```python
from build123d import *

# Parameters (mm, degrees)
F1_DEPTH = 5.08
F2_R     = 3.175
F4_DEPTH = 12.7
F5_W     = 14.224
F5_H     = 14.224
F6_DEPTH = 43.7134


with BuildPart() as f1:
    # F0 (on Front) → F1 (new body)
    with BuildSketch(Plane.XZ):
        with BuildLine():
            Line((9.525, 12.7), (-9.525, 12.7))
            ThreePointArc((-9.525, 12.7), (-11.770064, 11.770064), (-12.7, 9.525))
            Line((-12.7, 9.525), (-12.7, -9.525))
            ThreePointArc((-12.7, -9.525), (-11.770064, -11.770064), (-9.525, -12.7))
            Line((-9.525, -12.7), (9.525, -12.7))
            ThreePointArc((9.525, -12.7), (11.770064, -11.770064), (12.7, -9.525))
            Line((12.7, -9.525), (12.7, 9.525))
            ThreePointArc((12.7, 9.525), (11.770064, 11.770064), (9.525, 12.7))
        make_face()
    extrude(amount=F1_DEPTH)

    # F2
    f2_edges = [f1.edges().sort_by_distance(p)[0] for p in [
        (12.7, -5.08, 0),
    ]]
    fillet(f2_edges, radius=F2_R)

    # F3 (on face) → F4 (join)
    with BuildSketch(Plane(origin=(0, 0, 0), x_dir=(-1, 0, 0), z_dir=(0, 1, 0))):
        with BuildLine():
            ThreePointArc((9.652, 8.636), (9.35442, 9.35442), (8.636, 9.652))
            Line((8.636, 9.652), (-8.636, 9.652))
            ThreePointArc((-8.636, 9.652), (-9.35442, 9.35442), (-9.652, 8.636))
            Line((-9.652, 8.636), (-9.652, -8.636))
            ThreePointArc((-9.652, -8.636), (-9.35442, -9.35442), (-8.636, -9.652))
            Line((-8.636, -9.652), (8.636, -9.652))
            ThreePointArc((8.636, -9.652), (9.35442, -9.35442), (9.652, -8.636))
            Line((9.652, -8.636), (9.652, 8.636))
        make_face()
    extrude(amount=F4_DEPTH)

    # F5 (on face) → F6 (cut)
    with BuildSketch(Plane(origin=(0, 0, 0), x_dir=(-1, 0, 0), z_dir=(0, 1, 0))):
        Rectangle(F5_W, F5_H)
    extrude(amount=F6_DEPTH, mode=Mode.SUBTRACT)


solid = f1.part
```
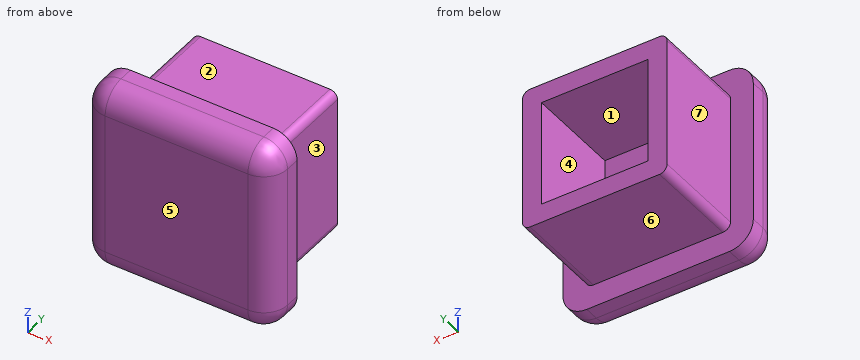
For this review, take the finished solid that the model builds, in its own axes (mm). Face numbers are marked on the shaded views. A direction names the side the tool comes from. Round coordinates to 2 decimals unless told otherwise and drop trailing zeros. Order: outer loops, then holes, each group sorted by start corner. A loop starts at its lowest first (then second) coordinate and runs counter-clockwise, first axis right, second up.
Q1. Insertion check: P1, Ø1.5, axis at x = -6, y = -3, coming from the -Z side; P2, Ø10, axis at y = 6.5, z = 1, coming from the -X side; P3, Ø4, axis at x = 2, y = 3.5, coming from the -Z side; P4, Ø12.5, axis at x = -1.5, z = 0, coming from the +Y side. Each pin has a flat end and moves straight along its axis. Give the tip position at first contact, or say it passes through.
Findings below:
P1: stops at z = -12.68
P2: stops at x = -9.65
P3: stops at z = -9.65
P4: stops at y = 12.7
Q2. We need section B-B, the plane x = -7.75. Give the boundary of the cut face in (y, z) (3 decimals).
Findings below:
outline: (-5.08, -9.525) arc R3.175 ccw to (-1.905, -12.7) - (0, -12.7) - (0, -9.652) - (12.7, -9.652) - (12.7, 9.652) - (0, 9.652) - (0, 12.7) - (-1.905, 12.7) arc R3.175 ccw to (-5.08, 9.525) - close
Q3. Mouldability with a two-part tool opening along X and no side actions: class the marked faces 1, 2 and 3 as pulls with the +X half, pulls with the -X half, needs draft (parallel to the pull), parting line crosses it, or undercut.
Findings below:
face 1: undercut
face 2: needs draft
face 3: pulls with the +X half
Q4. We need section A-A, the plane y = 5. Give the boundary of the cut face in (x, z), plus the area to 3 significant figures.
Findings below:
outline: (-9.65, -8.64) arc R1.02 ccw to (-8.64, -9.65) - (8.64, -9.65) arc R1.02 ccw to (9.65, -8.64) - (9.65, 8.64) arc R1.02 ccw to (8.64, 9.65) - (-8.64, 9.65) arc R1.02 ccw to (-9.65, 8.64) - close; hole (-7.11, -7.11) - (7.11, -7.11) - (7.11, 7.11) - (-7.11, 7.11) - close
area: 169 mm2
Q5. We need section D-D, the plane x = -2. Give the boundary of the cut face in (y, z) (3 decimals), plus the area to 3 significant figures.
Findings below:
outline: (-5.08, -9.525) arc R3.175 ccw to (-1.905, -12.7) - (0, -12.7) - (0, -9.652) - (12.7, -9.652) - (12.7, -7.112) - (0, -7.112) - (0, 7.112) - (12.7, 7.112) - (12.7, 9.652) - (0, 9.652) - (0, 12.7) - (-1.905, 12.7) arc R3.175 ccw to (-5.08, 9.525) - close
area: 189 mm2
Q6. We need section C-C, the plane z = 7.75. Give the boundary of the cut face in (x, y) (3 decimals), plus the area to 3 significant figures.
Findings below:
outline: (-12.7, -1.905) arc R3.175 ccw to (-9.525, -5.08) - (9.525, -5.08) arc R3.175 ccw to (12.7, -1.905) - (12.7, 0) - (9.652, 0) - (9.652, 12.7) - (-9.652, 12.7) - (-9.652, 0) - (-12.7, 0) - close
area: 370 mm2
Q7. Machinability: for the marked faces 4, 5, 6 and 7, which of the approach directions +Z, -Z, +X, -X, +Y, -Y give a long, thin tool a straight path to every point of the face, cutting with its end or side? Answer none if there is none.
Findings below:
face 4: +Y
face 5: +Z, -Z, +X, -X, -Y
face 6: -Z, +X, -X, +Y
face 7: +Z, -Z, -X, +Y
Q8. Wall thickness on line 1 (Z direction, x = -5, y = 2); line 2 (Y direction, x = 6.5, z = -5.75): over which ranges is each line inside the solid? List them lowest first.
Findings below:
line 1: z = -9.65 to -7.11, 7.11 to 9.65
line 2: y = -5.08 to 0
